Geometry check sheet. Reference: drawing and pictorial views, mm from the part's lowest x, y, z. A direction names the side the tool comes from. Round coordinates to 2 decimals unless told otherwise and drop trailing zeros. Order: outer loops, then holes, each group sorted by start corner. A loop starts at its lowest first (then second) coordinate and runs counter-clockwise, first axis right, second up. Notation, with made-up numbers: M 41.25,8 L 68.25,8 A15 cw 68.25,17 Z; hole C 80.5,27.25 d10. An arc over 180 degrees is marked long. Answer as a JSON object with one key per item and string values. Group by question number.
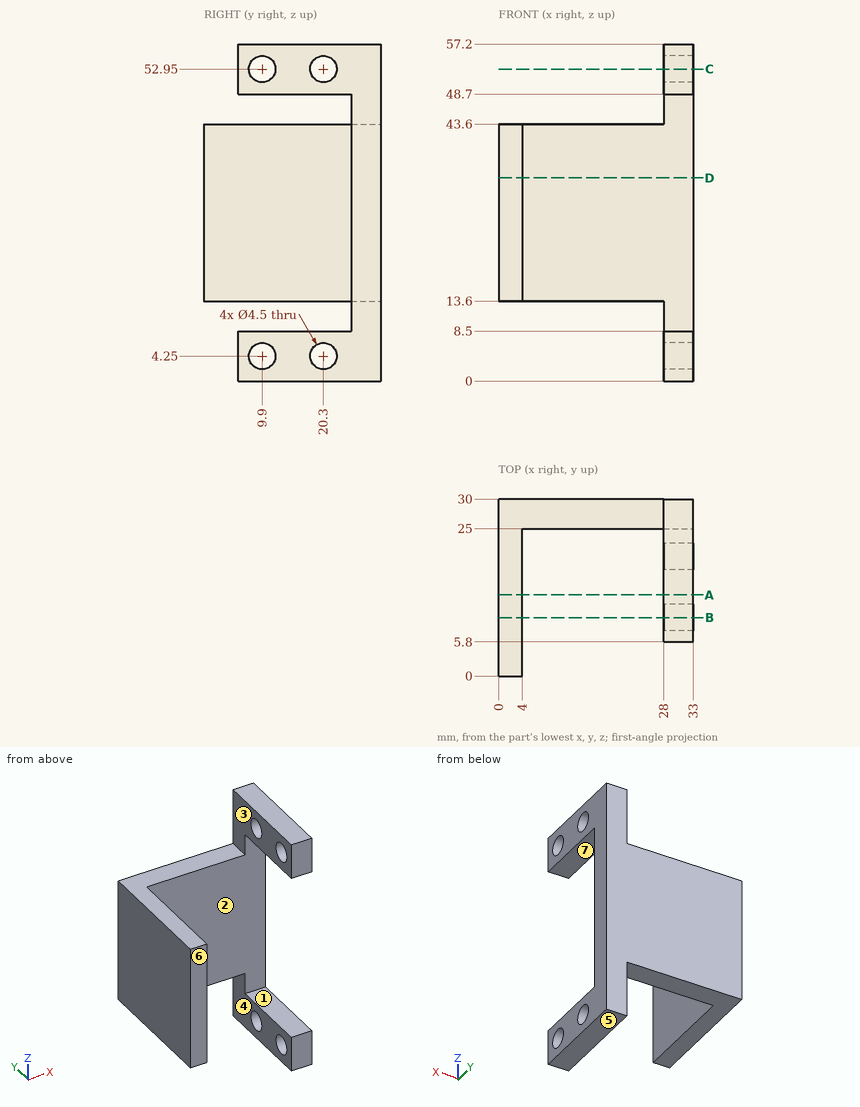
Q1. Tool access check on the marked faces 1, 2, 3 and 4. Record the directions out of +Z, -Z, +X, -X, +Y, -Y that give a thin tool (end or side, any length) a straight path to the whole face; none if there is none.
Q2. Cross-section at D-D, the plane z = 34.5. Record the cut outline in (x, y), then the cut area to 3 significant figures.
Q3. Cross-section at B-B, the plane y = 9.9. Record the cut outline in (x, z), then the cut area to 3 significant figures.
Q4. Cross-section at A-A, the plane y = 13.75. Record the cut outline in (x, z).
Q5. Cross-section at C-C, the plane z = 52.95. Record the cut outline in (x, y), then the cut area to 3 significant figures.
Q6. Gauge pin test, flat ends, axial feed: pin 1 Ø2.5 at (y, z) = (9.9, 4.25) entering from +X; pin 2 Ø6 at (x, z) = (20, 46) entering from -Y; pin 3 Ø4 at (y, z) = (23, 51.5) entering from -X; pin 4 Ø2.5 at (x, z) = (31.5, 51) entering from -Y. Record the tip position at first contact, or that the pin passes through.
Q7. Release check for a two-part mould opening along Z. For the marked faces 5, 6 and 7 record: released by +Z, released by -Z, zero draft, split by the parting line, or undercut.
Q8. Thickness scan on line 1 (Z direction, x = 29.5, y = 20.5); line 2 (Y direction, x = 29, z = 4); line 3 (X direction, y = 8.5, z = 28.5). Record the ranges inside material, lowest first. Write a range as from..to.
Conclusion:
{
 "1": {"face 1": "+X, -X, -Y", "face 2": "+X, -Y", "face 3": "+Z, -X, +Y, -Y", "face 4": "-Z, -X, +Y, -Y"},
 "2": {"outline": "M 0,0 L 4,0 L 4,25 L 33,25 L 33,30 L 0,30 Z", "area": "265 mm2"},
 "3": {"outline": "M 0,13.6 L 4,13.6 L 4,43.6 L 0,43.6 Z; M 28,0 L 33,0 L 33,2 L 28,2 Z; M 28,6.5 L 33,6.5 L 33,8.5 L 28,8.5 Z; M 28,48.7 L 33,48.7 L 33,50.7 L 28,50.7 Z; M 28,55.2 L 33,55.2 L 33,57.2 L 28,57.2 Z", "area": "160 mm2"},
 "4": {"outline": "M 0,13.6 L 4,13.6 L 4,43.6 L 0,43.6 Z; M 28,0 L 33,0 L 33,8.5 L 28,8.5 Z; M 28,48.7 L 33,48.7 L 33,57.2 L 28,57.2 Z"},
 "5": {"outline": "M 28,5.8 L 33,5.8 L 33,7.65 L 28,7.65 Z; M 28,12.15 L 33,12.15 L 33,18.05 L 28,18.05 Z; M 28,22.55 L 33,22.55 L 33,30 L 28,30 Z", "area": "76.0 mm2"},
 "6": {"pin 1": "through", "pin 2": "y = 25", "pin 3": "x = 28", "pin 4": "y = 5.8"},
 "7": {"face 5": "released by -Z", "face 6": "zero draft", "face 7": "undercut"},
 "8": {"line 1": "0..2.01, 6.49..8.5, 48.7..50.71, 55.19..57.2", "line 2": "5.8..7.66, 12.14..18.06, 22.54..30", "line 3": "0..4"}
}
